Autodesk Inventor part; units mm, degrees
ref_plane "Start Plane" through (0, 0, 0) normal (0, 0, 1) x (1, 0, 0)
ref_plane "End Plane" through (0, 0, 25.4) normal (0, 0, 1) x (1, 0, 0)
ref_plane "YZ Plane" through (0, 0, 0) normal (1, 0, 0) x (0, 1, 0)
ref_plane "Start Plane" through (0, 0, 0) normal (0, 0, 1) x (1, 0, 0)
ref_plane "End Plane" through (0, 0, 25.4) normal (0, 0, 1) x (1, 0, 0)
sketch "Sketch" plane through (0, 0, 0) normal (0, 0, 1) x (1, 0, 0)
  line L0 (-12.7, -25.4) -> (12.7, -25.4)
  line L1 (12.7, -25.4) -> (12.7, 25.4)
  line L2 (12.7, 25.4) -> (-12.7, 25.4)
  line L3 (-12.7, 25.4) -> (-12.7, -25.4)
  line L4 (-12.7, -25.4) -> (12.7, 25.4) construction
  line L5 (12.7, -25.4) -> (-12.7, 25.4) construction
  line L6 (-9.525, -22.225) -> (9.525, -22.225)
  line L7 (9.525, -22.225) -> (9.525, 22.225)
  line L8 (9.525, 22.225) -> (-9.525, 22.225)
  line L9 (-9.525, 22.225) -> (-9.525, -22.225)
  line L10 (-9.525, -22.225) -> (9.525, 22.225) construction
  line L11 (9.525, -22.225) -> (-9.525, 22.225) construction
  point P0 (0, 0)
  dimension "d0" = 25.4
  dimension "d1" = 50.8
  dimension "d2" = 3.175
  dimension "d3" = 3.175
extrude "Body" add sketch "Sketch" along normal up to surface (25.4 mm away) from surface at 0
sketch "Sketch6" plane through (0, 0, 0) normal (0, 0, 1) x (1, 0, 0)
  line L0 (0, 0) -> (10, 0)
ref_plane "Work Plane5" through (0, 0, 0) normal (0, -1, 0) x (1, 0, 0)
sketch "Sketch7" plane through (0, 0, 0) normal (0, -1, 0) x (1, 0, 0)
  line L0 (-2, 0) -> (12, 0)
  line L1 (-2, 25.4) -> (12, 25.4)
  dimension "d11" = 25.4
sketch "Sketch8" plane through (-12.7, -25.4, 25.4) normal (0, 0, 1) x (1, 0, 0)
  point P0 (12.7, 25.4)
equation "\"d0\" = Width"
equation "\"d1\" = Height"
equation "\"d2\" = Thickness"
equation "\"d3\" = Thickness"
equation "\"Height\" = 50.8"
equation "\"Width\" = 25.4"
equation "\"Thickness\" = 3.175"
equation "\"BaseLength\" = 25.4"
equation "\"G_OFFSET_START\" = 0"
equation "\"G_OFFSET_END\" = 0"
equation "\"d7\" = BaseLength + G_OFFSET_END"
equation "\"G_L\" = d11"
properties part number "AL RECT TUBE 2 x 1 x 0.125" material "Aluminum 6061"
For this review, take the finished solid that the model builds, in its own axes (mm). A direction names the side the tool comes from. Round coordinates to 2 decimals unless told otherwise and drop trailing zeros. Order: outer loops, then holes, each group sorted by start corner. A loop starts at its lowest first (then second) coordinate and runs counter-clockwise, first axis right, second up. Notation, with made-up numbers: M 68.25,26 L 121.25,26 A19 cw 121.25,55 Z; hole C 71.25,41 d3. An arc over 180 degrees is marked long. Use a Markdown table: item, result. Add a question column.
Item 1: Add section B-B, the plane x = -6.25. Give the boundary of the cut face in (y, z) (3 decimals).
Item 2: Tool access review of faces 1 (the flat face through (-10, -2, 0)), 2 (the flat face through (-9.525, 0, 13)): name each direction out of +Z, -Z, +X, -X, +Y, -Y from which nothing blocks a thin tool from reaching the whole face with its end or side.
Item 3: Add section A-A, the plane y = -20.5. Give the boundary of the cut face in (x, z) (3 decimals), then the cut area to 3 significant figures.
Item 4: Add section C-C, the plane z = 9.25. Give the boundary of the cut face in (x, y) (3 decimals), then the cut area to 3 significant figures.
Item 5: To check wall thickness, follow line 1 along X through (y, z) = (11, 12) (3 decimals); line 2 along Y through (x, z) = (-5.5, 12) (3 decimals). State the ranges of each line that lie inside material, in increasing order.
Item 6: Mouldability with a two-part tool opening along Y and no side actions: class faces 3 (the flat face through (0, -22.225, 13)), 4 (the flat face through (0, 25.4, 13)), 5 (the flat face through (-10, -2, 25.4)) as released by +Y, released by -Y, zero draft, split by the parting line, or undercut.
Geometry results:
| question | item | result |
|---|---|---|
| 1 | outline | M -25.4,0 L -22.225,0 L -22.225,25.4 L -25.4,25.4 Z; M 22.225,0 L 25.4,0 L 25.4,25.4 L 22.225,25.4 Z |
| 2 | face 1 | -Z, +X, -X, +Y, -Y |
| 2 | face 2 | +Z, -Z |
| 3 | outline | M -12.7,0 L -9.525,0 L -9.525,25.4 L -12.7,25.4 Z; M 9.525,0 L 12.7,0 L 12.7,25.4 L 9.525,25.4 Z |
| 3 | area | 161 mm² |
| 4 | outline | M -12.7,-25.4 L 12.7,-25.4 L 12.7,25.4 L -12.7,25.4 Z; hole M -9.525,-22.225 L 9.525,-22.225 L 9.525,22.225 L -9.525,22.225 Z |
| 4 | area | 444 mm² |
| 5 | line 1 | x = -12.7 to -9.525, 9.525 to 12.7 |
| 5 | line 2 | y = -25.4 to -22.225, 22.225 to 25.4 |
| 6 | face 3 | undercut |
| 6 | face 4 | released by +Y |
| 6 | face 5 | zero draft |
